The listing builds one solid part. Answer for the finished solid, in the listing's coordinates (mm). Face numbers are marked on the shaded views. Give positions to 0.01 mm unless a question says otherwise; leave off trailing zeros. Write each loop counter-clockwise with the first axis right and the second up, starting at its lowest first coordinate (ties: lowest second). Pieces come first, ordered by that corner, then holes. Notation, with made-up numbers: (29.5, 66.5) -> (43.5, 66.5) arc R22 ccw to (43.5, 88.5) -> close; hole circle Ø1 at (-1.5, -2). An arc over 180 degrees is marked (long way). Put each result on its own line as item: value. Start each with the question number.
1) Flat-ended cylindrical pins translate along their axes: pin 1 Ø1.5 at (x, z) = (-2, -5) entering from +Y; pin 2 Ø1.5 at (x, z) = (-2, 9.5) entering from -Y; pin 3 Ø6 at (x, z) = (1, 6) entering from +Y; pin 4 Ø2 at (y, z) = (-44, -14.5) entering from -X. Find the tip coordinate at first contact, or state that the pin passes through.
2) Find the intervals of material crossed by line 1 along Z through (x, y) = (-3.75, -76.2) (3 decimals); line 2 along Z through (x, y) = (-1.75, 50.8); line 3 along Y through (x, z) = (1, -1), in increasing order. Write a range as from..to.
3) A cutting plane is placed at A-A (x = 2.5). Write down the section's boundary in (y, z) (3 decimals).
4) A cutting plane is placed at C-C (y = 2). Write down the section's boundary in (x, z).
5) For a pull along Z with two mould halves and no side action, classify the marked faces 1, 2 and 3 as released by +Z, released by -Z, zero draft, split by the parting line, or undercut.
6) A cutting plane is placed at B-B (z = 0). Write down the section's boundary in (x, y) (3 decimals), then the cut area to 3 significant figures.
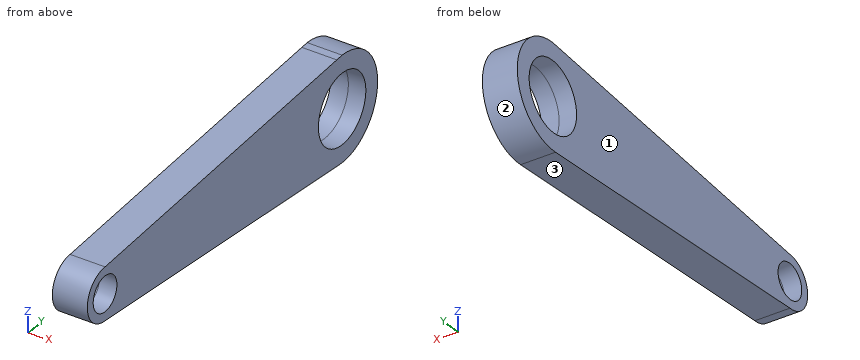
from build123d import *

# Parameters (mm, degrees)
F0_R     = 6.35
F1_DEPTH = 6.35


with BuildPart() as f1:
    # F0 (on Right) → F1 (new body, symmetric)
    with BuildSketch(Plane.YZ):
        with BuildLine():
            ThreePointArc((-76.2, -9.525), (-69.4648079092, -6.7351920908), (-66.675, 0))
            ThreePointArc((-66.675, 0), (-69.4648079092, 6.7351920908), (-76.2, 9.525))
            ThreePointArc((-76.2, 9.525), (-85.725, 0), (-76.2, -9.525))
        make_face()
        with Locations((-76.2, 0)):
            Circle(F0_R, mode=Mode.SUBTRACT)
        with BuildLine():
            ThreePointArc((-76.2, 9.525), (-69.4648079092, 6.7351920908), (-66.675, 0))
            Line((-66.675, 0), (31.75, 0))
            ThreePointArc((31.75, 0), (36.3598928544, 12.4252084741), (47.9584835301, 18.8368862648))
            Line((47.9584835301, 18.8368862648), (-76.2, 9.525))
        make_face()
        with BuildLine():
            Line((31.75, 0), (-66.675, 0))
            ThreePointArc((-66.675, 0), (-69.4648079092, -6.7351920908), (-76.2, -9.525))
            Line((-76.2, -9.525), (49.3672031886, -18.9960415165))
            ThreePointArc((49.3672031886, -18.9960415165), (36.8322285375, -12.9539129367), (31.75, 0))
        make_face()
        with BuildLine():
            ThreePointArc((47.9584835301, 18.8368862648), (36.3598928544, 12.4252084741), (31.75, 0))
            ThreePointArc((31.75, 0), (36.8322285375, -12.9539129367), (49.3672031886, -18.9960415165))
            ThreePointArc((49.3672031886, -18.9960415165), (63.7539129367, -13.9677714625), (69.85, 0))
            ThreePointArc((69.85, 0), (64.2703841816, 13.4703841816), (50.8, 19.05))
            Line((50.8, 19.05), (47.9584835301, 18.8368862648))
        make_face()
        with BuildLine():
            ThreePointArc((63.5, 0), (50.8, -12.7), (38.1, 0))
            ThreePointArc((38.1, 0), (50.8, 12.7), (63.5, 0))
        make_face(mode=Mode.SUBTRACT)
    extrude(amount=F1_DEPTH, both=True)


solid = f1.part
Reply:
1. pin 1: stops at y = 69.37
1. pin 2: stops at y = -79.96
1. pin 3: stops at y = 69.61
1. pin 4: passes through
2. line 1: z = -9.525..-6.35, 6.35..9.525
2. line 2: z = -19.05..-12.7, 12.7..19.05
2. line 3: y = -85.67..-82.47, -69.93..38.14, 63.46..69.82
3. outline: (-76.2, -9.525) -> (49.367, -18.996) arc R19.05 ccw (long way) to (50.8, 19.05) -> (-76.2, 9.525) arc R9.525 ccw to start; hole circle Ø12.7 at (-76.2, 0); hole circle Ø25.4 at (50.8, 0)
4. outline: (-6.35, -15.42) -> (6.35, -15.42) -> (6.35, 15.39) -> (-6.35, 15.39) -> close
5. face 1: zero draft
5. face 2: split by the parting line
5. face 3: released by -Z
6. outline: (-6.35, -85.725) -> (6.35, -85.725) -> (6.35, -82.55) -> (-6.35, -82.55) -> close; (-6.35, -69.85) -> (6.35, -69.85) -> (6.35, 38.1) -> (-6.35, 38.1) -> close; (-6.35, 63.5) -> (6.35, 63.5) -> (6.35, 69.85) -> (-6.35, 69.85) -> close
6. area: 1,490 mm2
